Check sheet for the modelled part. Datum: model origin and axes. Units: mm. Face numbers are marked on the shaded views. A direction names the side the tool comes from. Round coordinates to 2 decimals unless told otherwise and drop trailing zeros. Order: outer loops, then holes, each group sorted by start corner. A loop starts at its lowest first (then second) coordinate and runs counter-clockwise, first axis right, second up.
```python
from build123d import *

# Parameters (mm, degrees)
SKETCH1_W           = 3.175
SKETCH1_H           = 25.4
BOSS_EXTRUDE1_DEPTH = 38.1
FILLET1_R           = 2.54
SKETCH2_R           = 11.43
CUT_EXTRUDE1_DEPTH  = 38.1
SKETCH3_R           = 2.54
CUT_EXTRUDE3_DEPTH  = 61.989758362


with BuildPart() as part:
    # Sketch1 → Boss-Extrude1 (new body)
    with BuildSketch(Plane.XY):
        Polygon((0, 28.575), (0, 25.4), (3.175, 25.4), (38.1, 25.4), (38.1, 28.575), align=None)
        with Locations((1.5875, 12.7)):
            Rectangle(SKETCH1_W, SKETCH1_H)
    extrude(amount=BOSS_EXTRUDE1_DEPTH)

    # Fillet1
    fillet1_edges = [part.edges().sort_by_distance(p)[0] for p in [
        (0, 28.575, 19.05),
    ]]
    fillet(fillet1_edges, radius=FILLET1_R)

    # Sketch2 → Cut-Extrude1 (cut)
    with BuildSketch(Plane(origin=(0, 28.575, 0), x_dir=(1, 0, 0), z_dir=(0, 1, 0))):
        with Locations(Location((19.649884534, -19.05, 0), (0, 0, 270))):
            Circle(SKETCH2_R)
    extrude(amount=-CUT_EXTRUDE1_DEPTH, mode=Mode.SUBTRACT)

    # Sketch3 → Cut-Extrude3 (cut, through all)
    with BuildSketch(Plane.ZY):
        with Locations((7.62, 7.62)):
            Circle(SKETCH3_R)
        with Locations((30.48, 7.62)):
            Circle(SKETCH3_R)
    extrude(amount=-CUT_EXTRUDE3_DEPTH, mode=Mode.SUBTRACT)


solid = part.part
```
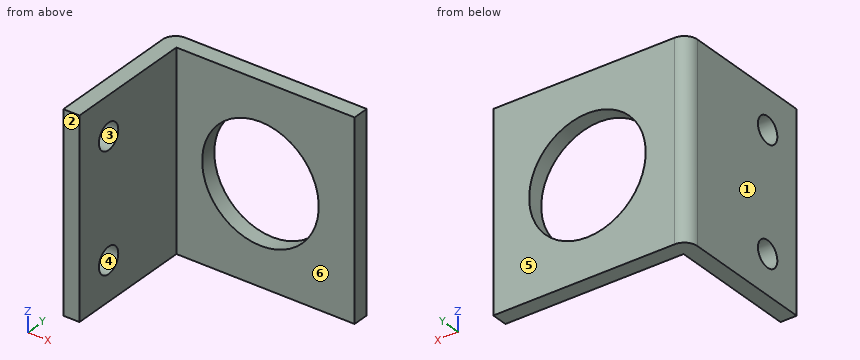
Item 1: Access from +Z, -Z, +X, -X, +Y, -Y to the whole of each face (thin tool, end or side, straight path). Record for the marked faces 5 and 6.
Answer:
face 5: +Z, -Z, +X, -X, +Y
face 6: +Z, -Z, +X, -Y
Item 2: Sectioned sample at C-C (x = 23). Record the cut outline in (y, z) (3 decimals), and give its area (3 significant figures).
Answer:
outline: (25.4, 0) - (28.575, 0) - (28.575, 8.122) - (25.4, 8.122) - close; (25.4, 29.978) - (28.575, 29.978) - (28.575, 38.1) - (25.4, 38.1) - close
area: 51.6 mm2
Item 3: Release check for a two-part mould opening along Y. For the marked faces 1, 2, 3 and 4 record: released by +Y, released by -Y, zero draft, split by the parting line, or undercut.
Answer:
face 1: zero draft
face 2: released by -Y
face 3: undercut
face 4: undercut
Item 4: Sectioned sample at D-D (z = 4). Record the cut outline in (x, y) (3 decimals).
Answer:
outline: (0, 0) - (3.175, 0) - (3.175, 25.4) - (38.1, 25.4) - (38.1, 28.575) - (2.54, 28.575) arc R2.54 ccw to (0, 26.035) - close
Item 5: Go/stop test with flat-tipped pins: P1, Ø1.5, axis at y = 12.5, z = 22.5, coming from the +X side (3 decimals); P2, Ø10.5, axis at x = 16, z = 26, coming from the -Y side. Record where each tip stops, or that it passes through.
Answer:
P1: stops at x = 3.175
P2: stops at y = 25.4
Item 6: Sectioned sample at A-A (z = 19.05). Record the cut outline in (x, y) (3 decimals), and give its area (3 significant figures).
Answer:
outline: (0, 0) - (3.175, 0) - (3.175, 25.4) - (8.22, 25.4) - (8.22, 28.575) - (2.54, 28.575) arc R2.54 ccw to (0, 26.035) - close; (31.08, 25.4) - (38.1, 25.4) - (38.1, 28.575) - (31.08, 28.575) - close
area: 128 mm2
Item 7: Sectioned sample at B-B (y = 7.62). Record the cut outline in (x, z) (3 decimals).
Answer:
outline: (0, 0) - (3.175, 0) - (3.175, 5.08) - (0, 5.08) - close; (0, 10.16) - (3.175, 10.16) - (3.175, 27.94) - (0, 27.94) - close; (0, 33.02) - (3.175, 33.02) - (3.175, 38.1) - (0, 38.1) - close
Item 8: Scan lines: line 1 along X through (y, z) = (19.25, 7.5) (3 decimals); line 2 along Y through (x, z) = (1, 7); line 3 along X through (y, z) = (26.6, 19.05). Record each from-to range of solid material in increasing order.
Answer:
line 1: x = 0 to 3.175
line 2: y = 0 to 5.16, 10.08 to 28.05
line 3: x = 0.06 to 8.22, 31.08 to 38.1
